Verification items for the finished model (mm, model axes). A direction names the side the tool comes from. Round coordinates to 2 decimals unless told otherwise and drop trailing zeros. Write each loop counter-clockwise with the first axis right and the second up, starting at its lowest first coordinate (ties: lowest second). Pieces come first, ordered by that corner, then holes.
from build123d import *

# Parameters (mm, degrees)
BOSS_EXTRUDE1_DEPTH = 10
BOSS_EXTRUDE3_DEPTH = 15


with BuildPart() as part:
    # Sketch1 → Boss-Extrude1 (new body)
    with BuildSketch(Plane.XY):
        with BuildLine():
            Line((-30, 0), (-30, 10))
            ThreePointArc((-30, 10), (-15, 25), (0, 10))
            Line((0, 10), (0, 0))
            Line((0, 0), (-30, 0))
        make_face()
    extrude(amount=BOSS_EXTRUDE1_DEPTH)

    # Sketch2 → Boss-Extrude3 (add)
    with BuildSketch(Plane.XY.offset(10)):
        with BuildLine():
            ThreePointArc((0, 25), (-10.055269439, 7.220988407), (-29.161787258, 0))
            Line((-29.161787258, 0), (0, 0))
            Line((0, 0), (0, 25))
        make_face()
    extrude(amount=BOSS_EXTRUDE3_DEPTH)


solid = part.part
Q1. Tool access check on faces 1 (the flat face through (-1, 18, 10)), 2 (the cylindrical face through (-9.835, 7.412, 17.395)), 3 (the cylindrical face through (-15, 25, 5)), 4 (the flat face through (0, 10, 15)). Record the directions out of +Z, -Z, +X, -X, +Y, -Y that give a thin tool (end or side, any length) a straight path to the whole face; none if there is none.
Recorded:
face 1: -Z, +X, +Y
face 2: +Z, -X, +Y
face 3: -Z, +Y
face 4: +Z, -Z, +X, +Y, -Y
Q2. Sectioned sample at A-A (y = 21.75). Enter the section's corners in (x, z), plus the area to 3 significant figures.
Recorded:
outline: (-24.32, 0) - (-5.68, 0) - (-5.68, 10) - (-24.32, 10) - close; (-0.74, 10) - (0, 10) - (0, 25) - (-0.74, 25) - close
area: 198 mm2
Q3. Material ranges on line 1 along Z through (x, y) = (-6.5, 20.75); line 2 along Y through (x, z) = (-4, 13); line 3 along X through (y, z) = (12.25, 5.75), recorded low to high.
Recorded:
line 1: z = 0 to 10
line 2: y = 0 to 14.32
line 3: x = -29.83 to -0.17
Q4. Sectioned sample at B-B (x = -16.5). Enter the section's corners in (y, z), plus the area to 3 significant figures.
Recorded:
outline: (0, 0) - (24.92, 0) - (24.92, 10) - (3, 10) - (3, 25) - (0, 25) - close
area: 294 mm2
Q5. Depth check by flat-ended pin: P1, Ø1, axis at y = 15.5, z = 14, coming from the -X side; P2, Ø2, axis at x = -23, y = 14.5, coming from the +Z side; P3, Ø1.7, axis at x = -1, y = 18.5, coming from the -Z side. Enter the tip coordinate at first touch or a pass-through.
Recorded:
P1: stops at x = -3.6
P2: stops at z = 10
P3: stops at z = 10
Q6. Sectioned sample at D-D (z = 19). Enter the section's corners in (x, y).
Recorded:
outline: (-29.16, 0) - (0, 0) - (0, 25) arc R30 cw to start
Q7. Sectioned sample at C-C (y = 16.75). Enter the section's corners in (x, z), plus the area to 3 significant figures.
Recorded:
outline: (-28.4, 0) - (-1.6, 0) - (-1.6, 10) - (0, 10) - (0, 25) - (-2.66, 25) - (-2.66, 10) - (-28.4, 10) - close
area: 308 mm2
